```python
from build123d import *

# Parameters (mm, degrees)
SKETCH2_R                   = 0.5
SKETCH2_W                   = 24
SKETCH2_H                   = 20
BASE_DEPTH                  = 4
FILLET1_R                   = 2
M3_CLEARANCE_HOLE1_REACH    = 70.374
M3_CLEARANCE_HOLE1_BORE_R   = 1.7
TAP_DRILL_FOR_M3X0_5_TAP1_D = 2.5
SKETCH10_R                  = 1.4
CUT_EXTRUDE1_DEPTH          = 10


with BuildPart() as part:
    # Sketch2 → Base (new, symmetric)
    with BuildSketch(Plane.XY):
        with BuildLine():
            Line((18, 0), (-18, 0))
            Line((-18, 0), (-18, 6.963574124))
            ThreePointArc((-18, 6.963574124), (-20.349128313, 15.023068249), (-26.660726074, 20.558190929))
            Line((-26.660726074, 20.558190929), (-56.290473047, 34.374768852))
            ThreePointArc((-56.290473047, 34.374768852), (-58.378054978, 39.313887584), (-53.676261446, 41.891877064))
            Line((-53.676261446, 41.891877064), (-13.708280328, 32.405461008))
            ThreePointArc((-13.708280328, 32.405461008), (-11.988094908, 32.101710083), (-10.244260752, 32))
            Line((-10.244260752, 32), (10.244260752, 32))
            ThreePointArc((10.244260752, 32), (11.988094908, 32.101710083), (13.708280328, 32.405461008))
            Line((13.708280328, 32.405461008), (53.676261446, 41.891877064))
            ThreePointArc((53.676261446, 41.891877064), (58.378054978, 39.313887584), (56.290473047, 34.374768852))
            Line((56.290473047, 34.374768852), (26.660726074, 20.558190929))
            ThreePointArc((26.660726074, 20.558190929), (20.349128313, 15.023068249), (18, 6.963574124))
            Line((18, 6.963574124), (18, 0))
        make_face()
        with Locations((-54.6, 38)):
            Circle(SKETCH2_R, mode=Mode.SUBTRACT)
        with Locations(Location((54.6, 38, 0), (0, 0, 180))):
            Circle(SKETCH2_R, mode=Mode.SUBTRACT)
        with Locations((-50.841229517, 36.631919427)):
            Circle(SKETCH2_R, mode=Mode.SUBTRACT)
        with Locations(Location((50.841229517, 36.631919427, 0), (0, 0, 180))):
            Circle(SKETCH2_R, mode=Mode.SUBTRACT)
        with Locations((0, 17)):
            Rectangle(SKETCH2_W, SKETCH2_H, mode=Mode.SUBTRACT)
        with BuildLine():
            Line((-20, 23.901748263), (-20, 29.23459547))
            ThreePointArc((-20, 29.23459547), (-20.430965495, 30.474809453), (-21.538130723, 31.180534002))
            Line((-21.538130723, 31.180534002), (-39.406838724, 35.421678882))
            ThreePointArc((-39.406838724, 35.421678882), (-42.426006691, 33.766271599), (-41.085505358, 30.594709734))
            Line((-41.085505358, 30.594709734), (-22.845236523, 22.089132689))
            ThreePointArc((-22.845236523, 22.089132689), (-20.925400783, 22.214965371), (-20, 23.901748263))
        make_face(mode=Mode.SUBTRACT)
        with BuildLine():
            Line((20, 23.901748263), (20, 29.23459547))
            ThreePointArc((20, 29.23459547), (20.430965495, 30.474809453), (21.538130723, 31.180534002))
            Line((21.538130723, 31.180534002), (39.406838724, 35.421678882))
            ThreePointArc((39.406838724, 35.421678882), (42.426006691, 33.766271599), (41.085505358, 30.594709734))
            Line((41.085505358, 30.594709734), (22.845236523, 22.089132689))
            ThreePointArc((22.845236523, 22.089132689), (20.925400783, 22.214965371), (20, 23.901748263))
        make_face(mode=Mode.SUBTRACT)
    extrude(amount=BASE_DEPTH, both=True)

    # Fillet1
    fillet1_edges = [part.edges().sort_by_distance(p)[0] for p in [
        (-12, 27, 0),
        (-12, 7, 0),
        (12, 7, 0),
        (12, 27, 0),
    ]]
    fillet(fillet1_edges, radius=FILLET1_R)

    # M3 Clearance Hole1 bore → M3 Clearance Hole1 (cut, up to next)
    with BuildSketch(Plane(origin=(0, 7, 0), x_dir=(1, 0, 0), z_dir=(0, 1, 0)), mode=Mode.PRIVATE) as m3_clearance_hole1_sk1:
        with Locations((-8, 0)):
            Circle(M3_CLEARANCE_HOLE1_BORE_R)
    m3_clearance_hole1_tool1 = extrude(m3_clearance_hole1_sk1.sketch, amount=-M3_CLEARANCE_HOLE1_REACH, mode=Mode.PRIVATE) & part.part
    # M3 Clearance Hole1 bore → M3 Clearance Hole1 (cut, up to next)
    with BuildSketch(Plane(origin=(0, 7, 0), x_dir=(1, 0, 0), z_dir=(0, 1, 0)), mode=Mode.PRIVATE) as m3_clearance_hole1_sk2:
        with Locations((8, 0)):
            Circle(M3_CLEARANCE_HOLE1_BORE_R)
    m3_clearance_hole1_tool2 = extrude(m3_clearance_hole1_sk2.sketch, amount=-M3_CLEARANCE_HOLE1_REACH, mode=Mode.PRIVATE) & part.part
    add(m3_clearance_hole1_tool1.solids().sort_by_distance((-8, 7, 0))[0], mode=Mode.SUBTRACT)
    add(m3_clearance_hole1_tool2.solids().sort_by_distance((8, 7, 0))[0], mode=Mode.SUBTRACT)

    # Tap Drill for M3x0.5 Tap1 (through all)
    with Locations(Plane.XY.offset(4)):
        with Locations((-54.6, 38), (54.6, 38), (-50.841229517, 36.631919427), (50.841229517, 36.631919427)):
            Hole(TAP_DRILL_FOR_M3X0_5_TAP1_D / 2)

    # Sketch10 → Cut-Extrude1 (cut)
    with BuildSketch(Plane(origin=(0, 32, 0), x_dir=(1, 0, 0), z_dir=(0, 1, 0))):
        with Locations(Location((-8, 0, 0), (0, 0, 270))):
            Circle(SKETCH10_R)
        with Locations(Location((8, 0, 0), (0, 0, 270))):
            Circle(SKETCH10_R)
    extrude(amount=-CUT_EXTRUDE1_DEPTH, mode=Mode.SUBTRACT)


solid = part.part
```
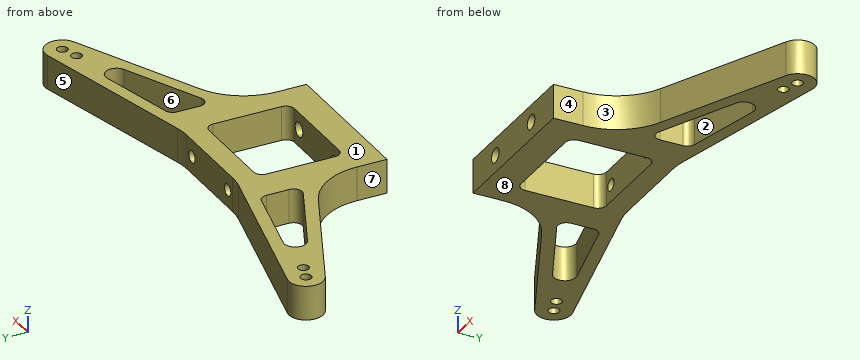
Build history of the part. All positions in model axes, mm. Face numbers are marked on the shaded views. A direction names the side the tool comes from. Round coordinates to 2 decimals unless told otherwise and drop trailing zeros. Write each loop counter-clockwise with the first axis right and the second up, starting at its lowest first coordinate (ties: lowest second). Pieces come first, ordered by that corner, then holes. Notation, with made-up numbers: (60.25, 36) -> (82.25, 36) arc R5 cw to (82.25, 41) -> close; hole circle Ø4 at (-3.5, -11). An arc over 180 degrees is marked (long way). Put each result on its own line as item: value.
Item 1: Slice it at C-C, the plane x = -47.5. Give the cut face in (y, z).
Here are the results:
outline: (30.28, -4) -> (40.43, -4) -> (40.43, 4) -> (30.28, 4) -> close
Item 2: Wall check: probe 1 along Y at (x, z) = (-4, -3); probe 2 along X at (y, z) = (4, -0.75); probe 3 along Z at (x, y) = (8, 3.75). Give the ranges that are in metal, low to high. Write a range as from..to.
Here are the results:
probe 1: y = 0..7, 27..32
probe 2: x = -18..-9.53, -6.47..6.47, 9.53..18
probe 3: z = -4..-1.7, 1.7..4
Item 3: Flat gauge pins, fed straight in: P1, Ø4, axis at y = 20.5, z = 0.5, coming from the -X side; P2, Ø1.5, axis at y = 25, z = 0, coming from the +X side; P3, Ø4, axis at x = 2, z = 2, coming from the -Y side; P4, Ø3, axis at y = 8, z = 0, coming from the +X side. Where does each tip first touch, or does it go through?
Here are the results:
P1: stops at x = -30.82
P2: stops at x = 37.79
P3: stops at y = 0
P4: stops at x = 18.22
Item 4: Tool access for the marked faces 4, 5, 6, 7 and 8: list every direction of +Z, -Z, +X, -X, +Y, -Y with a clear straight run to the whole face (end or side of a thin tool).
Here are the results:
face 4: +Z, -Z, +X, -Y
face 5: +Z, -Z, +Y
face 6: +Z, -Z
face 7: +Z, -Z, -X, -Y
face 8: -Z, +X, -X, +Y, -Y
Item 5: Slice it at B-B, the plane x = 15. Give the cut face in (y, z), plus the area to 3 significant figures.
Here are the results:
outline: (0, -4) -> (32.71, -4) -> (32.71, 4) -> (0, 4) -> close
area: 262 mm^2
Item 6: Two-plate mould, pull along X, no slides. Class the marked faces 1, 2 and 3: pulls with the +X half, pulls with the -X half, needs draft (parallel to the pull), parting line crosses it, or undercut.
Here are the results:
face 1: needs draft
face 2: undercut
face 3: pulls with the +X half
Item 7: Slice it at A-A, the plane x = 0.5. Give the cut face in (y, z), plus the area to 3 significant figures.
Here are the results:
outline: (0, -4) -> (7, -4) -> (7, 4) -> (0, 4) -> close; (27, -4) -> (32, -4) -> (32, 4) -> (27, 4) -> close
area: 96.0 mm^2
